```python
from build123d import *

# Parameters (mm, degrees)
SKETCH1_R           = 3.75
BOSS_EXTRUDE1_DEPTH = 7.5
SKETCH2_R           = 3.75
SKETCH2_R_2         = 2.5
CUT_EXTRUDE1_DEPTH  = 4
SKETCH3_R           = 1.65
BOSS_EXTRUDE2_DEPTH = 2


with BuildPart() as part:
    # Sketch1 → Boss-Extrude1 (new body)
    with BuildSketch(Plane(origin=(0, 0, 0), x_dir=(1, 0, 0), z_dir=(0, 1, 0))):
        Circle(SKETCH1_R)
    extrude(amount=BOSS_EXTRUDE1_DEPTH)

    # Sketch2 → Cut-Extrude1 (cut)
    with BuildSketch(Plane(origin=(0, 7.5, 0), x_dir=(1, 0, 0), z_dir=(0, 1, 0))):
        Circle(SKETCH2_R)
        Circle(SKETCH2_R_2, mode=Mode.SUBTRACT)
    extrude(amount=-CUT_EXTRUDE1_DEPTH, mode=Mode.SUBTRACT)

    # Sketch3 → Boss-Extrude2 (add)
    with BuildSketch(Plane(origin=(0, 7.5, 0), x_dir=(1, 0, 0), z_dir=(0, 1, 0))):
        Circle(SKETCH3_R)
    extrude(amount=BOSS_EXTRUDE2_DEPTH)


solid = part.part
```
Build history of the part. All positions in model axes, mm. A direction names the side the tool comes from. Round coordinates to 2 decimals unless told otherwise and drop trailing zeros. Write each loop counter-clockwise with the first axis right and the second up, starting at its lowest first coordinate (ties: lowest second). Pieces come first, ordered by that corner, then holes. Notation, with made-up numbers: (-39, -40) -> (-19, -40) arc R29 cw to (-19, -6) -> close; hole circle Ø5 at (36.25, -21). An arc over 180 degrees is marked (long way). Put each result on its own line as item: value.
Item 1: Tool access for faces 1 (the face through (0, 0, 0)), 2 (the face through (-1.216, 8.486, -1.115)): list every direction of +Z, -Z, +X, -X, +Y, -Y with a clear straight run to the whole face (end or side of a thin tool).
Here are the results:
face 1: +Z, -Z, +X, -X, -Y
face 2: +Y
Item 2: Wall check: probe 1 along X at (y, z) = (7, 0); probe 2 along Y at (x, z) = (-1.5, -2.75); probe 3 along Y at (x, z) = (2, 0). Give the ranges that are in metal, low to high. Write a range as from..to.
Here are the results:
probe 1: x = -2.5..2.5
probe 2: y = 0..3.5
probe 3: y = 0..7.5
Item 3: Slice it at A-A, the plane x = 0. Give the cut face in (y, z).
Here are the results:
outline: (0, -3.75) -> (3.5, -3.75) -> (3.5, -2.5) -> (7.5, -2.5) -> (7.5, -1.65) -> (9.5, -1.65) -> (9.5, 1.65) -> (7.5, 1.65) -> (7.5, 2.5) -> (3.5, 2.5) -> (3.5, 3.75) -> (0, 3.75) -> close
Item 4: Flat gauge pin, fed straight in: P1, Ø4, axis at y = 4.5, z = 0, coming from the +X side. Where does the tip first touch, or does it go through?
Here are the results:
P1: stops at x = 3.75
Item 5: Slice it at B-B, the plane z = 0. Give the cut face in (x, y).
Here are the results:
outline: (-3.75, 0) -> (3.75, 0) -> (3.75, 3.5) -> (2.5, 3.5) -> (2.5, 7.5) -> (1.65, 7.5) -> (1.65, 9.5) -> (-1.65, 9.5) -> (-1.65, 7.5) -> (-2.5, 7.5) -> (-2.5, 3.5) -> (-3.75, 3.5) -> close
Item 6: Slice it at C-C, the plane y = 0.5. Give the cut face in (x, z).
Here are the results:
outline: circle Ø7.5 at (0, 0)
Item 7: Slice it at D-D, the plane z = 2.25. Give the cut face in (x, y), plus the area to 3 significant figures.
Here are the results:
outline: (-3, 0) -> (3, 0) -> (3, 3.5) -> (1.09, 3.5) -> (1.09, 7.5) -> (-1.09, 7.5) -> (-1.09, 3.5) -> (-3, 3.5) -> close
area: 29.7 mm^2
